```python
from build123d import *

# Parameters (mm, degrees)
SKETCH1_W                = 157.48
SKETCH1_H                = 50.8
BOSS_EXTRUDE1_DEPTH      = 40.64
SKETCH37_W               = 81.28
SKETCH37_H               = 25.4
CUT_EXTRUDE32_DEPTH      = 171.388379885
BOSS_EXTRUDE5_DEPTH      = 25.4
CUT_EXTRUDE54_DEPTH      = 105.109019782
CUT_EXTRUDE54_DEPTH_BACK = 105.109019782
SKETCH45_W               = 63.5
SKETCH45_H               = 28.09875
SKETCH97_W               = 20.4891
SKETCH97_H               = 81.28
CUT_EXTRUDE72_DEPTH      = 44.45
SKETCH98_R               = 3.429
CUT_EXTRUDE73_DEPTH      = 102.162495521
SKETCH99_W               = 57.15
SKETCH99_H               = 38.1
CUT_EXTRUDE74_DEPTH      = 105.109019782
SKETCH101_W              = 6.35
SKETCH101_H              = 6.35
BOSS_EXTRUDE7_DEPTH      = 5.3975
BOSS_EXTRUDE8_REACH      = 106.109
SKETCH102_W              = 20.4891
SKETCH102_H              = 6.35
SKETCH103_R              = 3.429
CUT_EXTRUDE75_DEPTH      = 126.672259469


with BuildPart() as part:
    # Sketch1 → Boss-Extrude1 (new, symmetric)
    with BuildSketch(Plane.XY):
        with Locations((2.54, -25.4)):
            Rectangle(SKETCH1_W, SKETCH1_H)
    extrude(amount=BOSS_EXTRUDE1_DEPTH, both=True)

    # Sketch2 → Cut-Revolve1 (revolve, cut)
    with BuildSketch(Plane.XY, mode=Mode.PRIVATE) as cut_revolve1_sk:
        Polygon((-49.3609, 8.636), (-49.3609, -12.7), (-76.2, -12.7), (-76.2, -25.4), (19.629439755, -25.4), (72.533481331, -25.4), (72.533481331, -15.494), (47.133481331, -15.494), (47.133481331, 5.461390138), (4.437328256, 5.461390138), (4.4871, 8.636), align=None)
    revolve(cut_revolve1_sk.sketch.rotate(Axis((-607.361866059, -25.4, 0), (1, 0, 0)), 90), axis=Axis((-607.361866059, -25.4, 0), (1, 0, 0)), mode=Mode.SUBTRACT)

    # Sketch37 → Cut-Extrude32 (cut, through all)
    with BuildSketch(Plane(origin=(81.28, 0, 0), x_dir=(0, 0, -1), z_dir=(1, 0, 0))):
        with Locations((0, -12.7)):
            Rectangle(SKETCH37_W, SKETCH37_H)
    extrude(amount=-CUT_EXTRUDE32_DEPTH, mode=Mode.SUBTRACT)

    # Sketch39 → Boss-Extrude5 (add)
    with BuildSketch(Plane(origin=(0, -25.4, 0), x_dir=(1, 0, 0), z_dir=(0, 1, 0))):
        Polygon((-49.3609, -12.7), (-76.2, -12.7), (-76.2, -40.64), (81.28, -40.64), (81.28, 40.64), (-76.2, 40.64), (-76.2, 12.7), (-49.3609, 12.7), (-49.3609, 34.036), (4.4871, 34.036), (4.437328256, 30.861390138), (47.133481331, 30.861390138), (47.133481331, 9.906), (72.533481331, 9.906), (72.533481331, -9.906), (47.133481331, -9.906), (47.133481331, -30.861390138), (4.437328256, -30.861390138), (4.4871, -34.036), (-49.3609, -34.036), align=None)
    extrude(amount=BOSS_EXTRUDE5_DEPTH)

    # Sketch45 → Cut-Extrude54 (cut, two sides: drawn at the far end of the back side and taken through both)
    with BuildSketch(Plane.XY.offset(-CUT_EXTRUDE54_DEPTH_BACK)):
        with Locations((49.53, -14.049375)):
            Rectangle(SKETCH45_W, SKETCH45_H)
    extrude(amount=CUT_EXTRUDE54_DEPTH + CUT_EXTRUDE54_DEPTH_BACK, mode=Mode.SUBTRACT)

    # Sketch97 → Cut-Extrude72 (cut)
    with BuildSketch(Plane(origin=(0, 0, 0), x_dir=(1, 0, 0), z_dir=(0, 1, 0))):
        with Locations((-65.95545, 0)):
            Rectangle(SKETCH97_W, SKETCH97_H)
    extrude(amount=-CUT_EXTRUDE72_DEPTH, mode=Mode.SUBTRACT)

    # Sketch98 → Cut-Extrude73 (cut, through all)
    with BuildSketch(Plane(origin=(0, -44.45, 0), x_dir=(1, 0, 0), z_dir=(0, 1, 0))):
        with Locations(Location((-69.85, 25.4, 0), (0, 0, 270))):
            Circle(SKETCH98_R)
        with Locations(Location((-69.85, 12.7, 0), (0, 0, 270))):
            Circle(SKETCH98_R)
        with Locations(Location((-69.85, 0, 0), (0, 0, 270))):
            Circle(SKETCH98_R)
        with Locations(Location((-69.85, -12.7, 0), (0, 0, 270))):
            Circle(SKETCH98_R)
        with Locations(Location((-69.85, -25.4, 0), (0, 0, 270))):
            Circle(SKETCH98_R)
    extrude(amount=-CUT_EXTRUDE73_DEPTH, mode=Mode.SUBTRACT)

    # Sketch99 → Cut-Extrude74 (cut, through all)
    with BuildSketch(Plane(origin=(0, 0, 0), x_dir=(1, 0, 0), z_dir=(0, 1, 0))):
        with Locations((46.355, 0)):
            Rectangle(SKETCH99_W, SKETCH99_H)
    extrude(amount=-CUT_EXTRUDE74_DEPTH, mode=Mode.SUBTRACT)

    # Sketch101 → Boss-Extrude7 (add)
    with BuildSketch(Plane(origin=(0, -28.09875, 0), x_dir=(1, 0, 0), z_dir=(0, 1, 0))):
        with Locations((52.705, 22.225)):
            Rectangle(SKETCH101_W, SKETCH101_H)
        with Locations((65.405, 22.225)):
            Rectangle(SKETCH101_W, SKETCH101_H)
        with Locations((78.105, 22.225)):
            Rectangle(SKETCH101_W, SKETCH101_H)
        with Locations((78.105, -22.225)):
            Rectangle(SKETCH101_W, SKETCH101_H)
        with Locations((65.405, -22.225)):
            Rectangle(SKETCH101_W, SKETCH101_H)
        with Locations((52.705, -22.225)):
            Rectangle(SKETCH101_W, SKETCH101_H)
    extrude(amount=BOSS_EXTRUDE7_DEPTH)

    # Sketch102 → Boss-Extrude8 (add, up to next)
    with BuildSketch(Plane(origin=(0, 0, 0), x_dir=(1, 0, 0), z_dir=(0, 1, 0)), mode=Mode.PRIVATE) as boss_extrude8_sk1:
        with Locations((-65.95545, 37.465)):
            Rectangle(SKETCH102_W, SKETCH102_H)
    boss_extrude8_tool1 = extrude(boss_extrude8_sk1.sketch, amount=-BOSS_EXTRUDE8_REACH, mode=Mode.PRIVATE) - part.part
    # Sketch102 → Boss-Extrude8 (add, up to next)
    with BuildSketch(Plane(origin=(0, 0, 0), x_dir=(1, 0, 0), z_dir=(0, 1, 0)), mode=Mode.PRIVATE) as boss_extrude8_sk2:
        with Locations((-65.95545, -37.465)):
            Rectangle(SKETCH102_W, SKETCH102_H)
    boss_extrude8_tool2 = extrude(boss_extrude8_sk2.sketch, amount=-BOSS_EXTRUDE8_REACH, mode=Mode.PRIVATE) - part.part
    add(boss_extrude8_tool1.solids().sort_by_distance((-65.95545, 0, -37.465))[0])
    add(boss_extrude8_tool2.solids().sort_by_distance((-65.95545, 0, 37.465))[0])

    # Sketch103 → Cut-Extrude75 (cut, through all)
    with BuildSketch(Plane.XY.offset(40.64)):
        with Locations((-69.85, -6.35)):
            Circle(SKETCH103_R)
        with Locations((-69.85, -19.05)):
            Circle(SKETCH103_R)
        with Locations((-69.85, -31.75)):
            Circle(SKETCH103_R)
    extrude(amount=-CUT_EXTRUDE75_DEPTH, mode=Mode.SUBTRACT)


solid = part.part
```
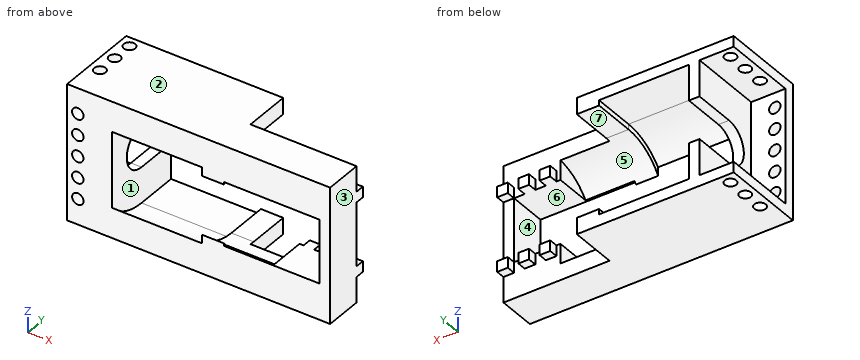
Design review of the part built by this model. Coordinates are the model's own, in mm. Face numbers are marked on the shaded views. A direction names the side the tool comes from. Round coordinates to 2 decimals unless told otherwise and drop trailing zeros. Order: outer loops, then holes, each group sorted by start corner. A loop starts at its lowest first (then second) coordinate and runs counter-clockwise, first axis right, second up. Notation, with made-up numbers: (72.25, 5) - (126.25, 5) arc R21 cw to (126.25, 35) - close; hole circle Ø4 at (6.5, -14.5). An arc over 180 degrees is marked (long way). Return JSON: item names as keys, results as strings.
Q1. Consider section D-D on x = -64. Write out the cut boundary in (y, z), plus the area to 3 significant figures.
Computed values:
{"outline": "(-50.8, -40.64) - (0, -40.64) - (0, -34.29) - (-44.45, -34.29) - (-44.45, 34.29) - (0, 34.29) - (0, 40.64) - (-50.8, 40.64) - close", "area": "1,080 mm2"}
Q2. Wall thickness on L1, parallel to Y at x = -69.85, z = 38; L2, parallel to X at y = -26.5, z = -22.5; L3, parallel to X at y = -35.5, z = -15: over which ranges is each line inside the solid? List them lowest first. Write a range as [from, to].
Computed values:
{"L1": "y = [-50.8, -35.18], [-28.32, -22.48], [-15.62, -9.78], [-2.92, 0]", "L2": "x = [-55.71, -49.36], [49.53, 55.88], [62.23, 68.58], [74.93, 81.28]", "L3": "x = [-55.71, -49.36], [74.93, 81.28]"}
Q3. For pin 1 Ø11 at (y, z) = (-19.5, 37) entering from +X; pin 2 Ø2.5 at (x, y) = (78, -26.5) entering from -Z; pin 3 Ø6 at (x, y) = (53, -26.5) entering from +Z; pin 4 Ø17.5 at (x, z) = (37.5, 29.5) entering from +Y, all flat-tipped, find the tip position at first contact; note any pin that passes through.
Computed values:
{"pin 1": "stops at x = 17.78", "pin 2": "stops at z = -25.4", "pin 3": "stops at z = 40.64", "pin 4": "stops at y = -28.1"}
Q4. Consider section B-B on y = -19.05. Write out the cut boundary in (x, z).
Computed values:
{"outline": "(-76.2, -40.64) - (-73.28, -40.64) - (-73.28, -34.29) - (-76.2, -34.29) - close; (-76.2, 34.29) - (-73.28, 34.29) - (-73.28, 40.64) - (-76.2, 40.64) - close; (-66.42, -40.64) - (17.78, -40.64) - (17.78, -30.86) - (4.44, -30.86) - (4.49, -34.04) - (-49.36, -34.04) - (-49.36, -12.7) - (-55.71, -12.7) - (-55.71, -34.29) - (-66.42, -34.29) - close; (-66.42, 34.29) - (-55.71, 34.29) - (-55.71, 12.7) - (-49.36, 12.7) - (-49.36, 34.04) - (4.49, 34.04) - (4.44, 30.86) - (17.78, 30.86) - (17.78, 40.64) - (-66.42, 40.64) - close"}
Q5. Consider section A-A on x = -20.5. Write out the cut boundary in (y, z), plus the area to 3 significant figures.
Computed values:
{"outline": "(-50.8, -40.64) - (0, -40.64) - (0, -34.04) - (-25.4, -34.04) arc R34.04 cw to (-50.8, -22.66) - close; (-50.8, 22.66) arc R34.04 cw to (-25.4, 34.04) - (0, 34.04) - (0, 40.64) - (-50.8, 40.64) - close", "area": "849 mm2"}
Q6. Machinability: for the marked faces 5, 6 and 7, which of the approach directions +Z, -Z, +X, -X, +Y, -Y give a long, thin tool a straight path to every point of the face, cutting with its end or side? Answer none if there is none.
Computed values:
{"face 5": "+Y", "face 6": "+Y, -Y", "face 7": "+X, +Y"}
Q7. The part is to be moulded in two halves that separate along X. For the marked faces 1, 2, 3 and 4, say which applies: pulls with the +X half, pulls with the -X half, needs draft (parallel to the pull), parting line crosses it, or undercut.
Computed values:
{"face 1": "undercut", "face 2": "needs draft", "face 3": "pulls with the +X half", "face 4": "undercut"}
Q8. Consider section C-C on z = 5.5. Write out the cut boundary in (x, y).
Computed values:
{"outline": "(-76.2, -50.8) - (-49.36, -50.8) - (-49.36, -36.85) - (-55.71, -36.85) - (-55.71, -44.45) - (-76.2, -44.45) - close; (74.93, -50.8) - (81.28, -50.8) - (81.28, -28.1) - (74.93, -28.1) - close"}
